Check sheet for the drawn part. Datum: minimum x, y, z corner. Units: mm. Give positions to 0.01 mm unless a question says otherwise; leave off trailing zeros. Order: outer loops, then holes, each group sorted by start corner. A loop starts at its lowest first (then second) coordinate and runs counter-clockwise, first axis right, second up.
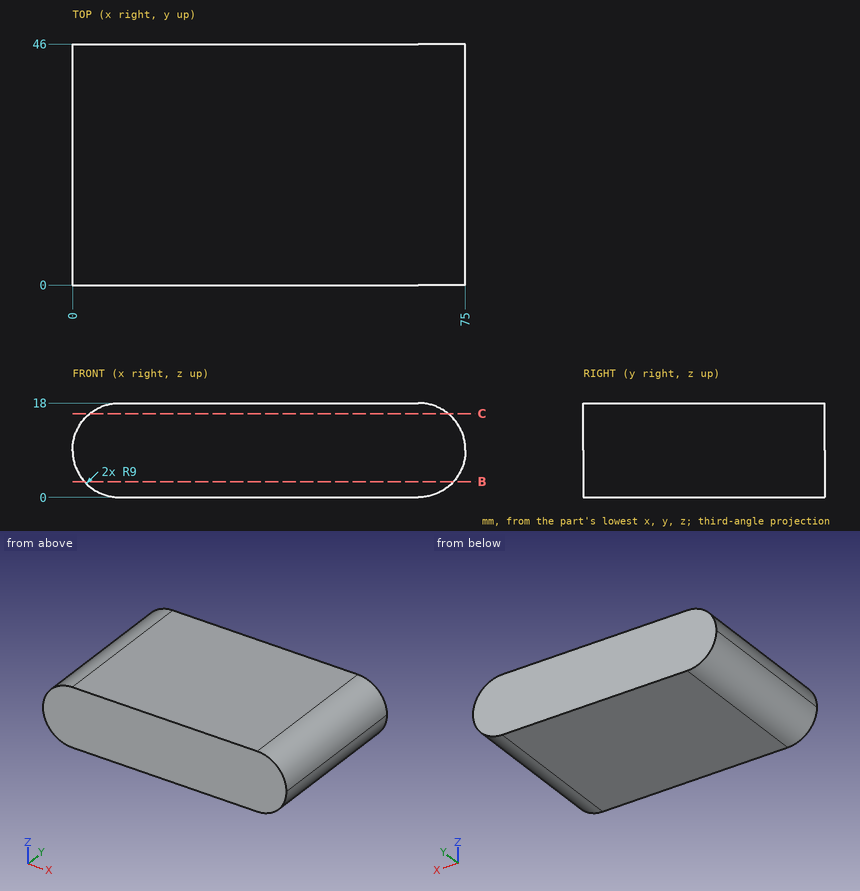
Item 1: Sectioned sample at C-C (z = 16). Enter the section's corners in (x, y), and give its area (3 significant figures).
Reported:
outline: (3.34, 0) - (71.66, 0) - (71.66, 46) - (3.34, 46) - close
area: 3,140 mm2
Item 2: Scan lines: L1, parallel to X at y = 15.5, z = 9.5; L2, parallel to X at y = 11.5, z = 1.5 (3 decimals); L3, parallel to Z at x = 6, y = 31.5. Record each from-to range of solid material in increasing order.
Reported:
L1: x = 0.01 to 74.99
L2: x = 4.025 to 70.975
L3: z = 0.51 to 17.49
Item 3: Gauge pin test, flat end, axial feed: pin 1 (6 mm diameter, centred on y = 39, z = 15, fed in from +X). Record the tip position at first contact, or that the pin passes through.
Reported:
pin 1: stops at x = 74.49
Item 4: Sectioned sample at B-B (z = 3). Enter the section's corners in (x, y).
Reported:
outline: (2.29, 0) - (72.71, 0) - (72.71, 46) - (2.29, 46) - close
